Autodesk Inventor part; units mm, degrees
ref_plane "YZ Plane" through (0, 0, 0) normal (1, 0, 0) x (0, 1, 0)
ref_plane "XZ Plane" through (0, 0, 0) normal (0, 1, 0) x (-1, 0, 0)
ref_plane "XY Plane" through (0, 0, 0) normal (0, 0, 1) x (1, 0, 0)
sketch "Sketch1" plane through (0, 0, 0) normal (0, 1, 0) x (-1, 0, 0)
  line L0 (101.6, 38.1) -> (-101.6, 38.1) construction
  line L1 (-101.6, 38.1) -> (-101.6, -38.1) construction
  line L2 (-101.6, -38.1) -> (101.6, -38.1) construction
  line L3 (101.6, -38.1) -> (101.6, 38.1) construction
  line L4 (101.6, 38.1) -> (-101.6, -38.1) construction
  line L5 (-101.6, 38.1) -> (101.6, -38.1) construction
  line L6 (-28.575, 66.675) -> (28.575, 66.675) construction
  line L7 (28.575, 66.675) -> (28.575, 9.525)
  line L8 (28.575, 9.525) -> (-28.575, 9.525) construction
  line L9 (-28.575, 9.525) -> (-28.575, 66.675)
  line L10 (-28.575, 66.675) -> (28.575, 9.525) construction
  line L11 (28.575, 66.675) -> (-28.575, 9.525) construction
  circle A0 centre (-38.1, 50.8) radius 3.175
  line L12 (0, 38.1) -> (0, -38.1) construction
  circle A1 centre (-38.1, 50.8) radius 9.525
  line L13 (-38.1, 60.325) -> (-28.575, 60.325)
  circle A2 centre (38.1, 50.8) radius 3.175
  circle A3 centre (38.1, 50.8) radius 9.525
  line L14 (38.1, 60.325) -> (28.575, 60.325)
  circle A4 centre (-76.2, -38.1) radius 1.7526
  circle A5 centre (-95.25, 3.175) radius 1.7526
  circle A6 centre (76.2, -38.1) radius 1.7526
  circle A7 centre (95.25, 3.175) radius 1.7526
  line L15 (-101.6, -38.1) -> (-101.6, 6.35)
  line L16 (-101.6, 6.35) -> (-44.4797, 57.8728)
  line L17 (101.6, -38.1) -> (101.6, 6.35)
  line L18 (101.6, 6.35) -> (44.4797, 57.8728)
  line L19 (-42.6417, 42.4275) -> (-87.975, 1.5367) construction
  line L20 (-87.975, 1.5367) -> (-87.975, -38.1)
  line L21 (87.975, -38.1) -> (87.975, 1.5367)
  line L22 (87.975, 1.5367) -> (42.6417, 42.4275) construction
  line L23 (0, -38.1) -> (-95.25, -38.1) construction
  line L24 (0, -38.1) -> (95.25, -38.1) construction
  circle A8 centre (-60.325, 35.0287) radius 1.7526
  circle A9 centre (-33.3375, 31.75) radius 1.7526
  line L25 (-38.1, 0) -> (-38.1, 41.275)
  line L26 (-38.1, 0) -> (0, 0) construction
  circle A10 centre (60.325, 35.0287) radius 1.7526
  circle A11 centre (33.3375, 31.75) radius 1.7526
  line L27 (38.1, 0) -> (38.1, 41.275)
  line L28 (38.1, 0) -> (0, 0) construction
  line L29 (-87.975, 0) -> (-65.115, 0)
  line L30 (-65.115, 0) -> (-65.115, -31.75)
  line L31 (-65.115, -31.75) -> (-87.975, -31.75)
  line L32 (-101.6, -38.1) -> (101.6, -38.1) construction
  line L33 (101.6, -38.1) -> (101.6, 19.05)
  line L34 (101.6, 19.05) -> (-101.6, 19.05) construction
  line L35 (-101.6, 19.05) -> (-101.6, -38.1)
  line L36 (-101.6, 19.05) -> (-87.5203, 19.05) construction
  line L37 (87.5203, 19.05) -> (101.6, 19.05) construction
  circle A12 centre (-38.1, 0) radius 3.175 construction
  circle A13 centre (-38.1, 0) radius 6.35 construction
  circle A14 centre (38.1, 0) radius 3.175 construction
  circle A15 centre (38.1, 0) radius 6.35 construction
  circle A16 centre (28.575, 9.525) radius 1.7526
  circle A17 centre (28.575, 9.525) radius 4.7625
  arc A18 (17.0773, 9.525) -> (28.575, 21.0227) centre (17.0773, 21.0227) ccw
  circle A19 centre (-28.575, 9.525) radius 1.7526
  circle A20 centre (-28.575, 9.525) radius 4.7625
  arc A21 (-28.575, 21.0227) -> (-17.0773, 9.525) centre (-17.0773, 21.0227) ccw
  arc A22 (31.4325, 5.715) -> (38.1, 19.05) centre (21.4312, 19.05) ccw
  arc A23 (-38.1, 19.05) -> (-31.4325, 5.715) centre (-21.4312, 19.05) ccw
  line L38 (-61.94, -38.1) -> (-61.94, 25.0204)
  line L39 (87.975, 0) -> (65.115, 0)
  line L40 (65.115, 0) -> (65.115, -31.75)
  line L41 (65.115, -31.75) -> (87.975, -31.75)
  line L42 (61.94, -38.1) -> (61.94, 25.0204)
  line L43 (-28.575, 4.7625) -> (28.575, 4.7625)
  line L44 (101.6, -31.75) -> (-101.6, -31.75)
  line L45 (-101.6, -31.75) -> (-101.6, -44.45) construction
  line L46 (-101.6, -44.45) -> (101.6, -44.45)
  line L47 (101.6, -44.45) -> (101.6, -31.75) construction
  circle A24 centre (0, -38.1) radius 1.7526
  circle A25 centre (38.1, -38.1) radius 1.7526
  circle A26 centre (-38.1, -38.1) radius 1.7526
  line L48 (101.6, -38.1) -> (76.2, -44.45)
  line L49 (-101.6, -38.1) -> (-76.2, -44.45)
  line L50 (76.2, -38.1) -> (76.2, -44.45) construction
  line L51 (-76.2, -38.1) -> (-76.2, -44.45) construction
  line L52 (59.1924, 41.2769) -> (32.488, 36.4361)
  circle A27 centre (60.325, 35.0287) radius 6.35
  circle A28 centre (33.3375, 31.75) radius 4.7625
  line L53 (-59.1924, 41.2769) -> (-32.488, 36.4361)
  circle A29 centre (-60.325, 35.0287) radius 6.35
  circle A30 centre (-33.3375, 31.75) radius 4.7625
  line L54 (-87.975, 0) -> (-65.115, 0)
  line L55 (-65.115, 0) -> (-65.115, -3.175)
  line L56 (-65.115, -3.175) -> (-87.975, -3.175)
  line L57 (-87.975, -3.175) -> (-87.975, 0)
  line L58 (-65.115, -15.875) -> (-87.975, -15.875) construction
  line L59 (-65.115, -28.575) -> (-87.975, -28.575)
  line L60 (-84.8, -38.1) -> (-84.8, 0.1248)
  line L61 (65.115, -3.175) -> (87.975, -3.175)
  line L62 (65.115, -15.875) -> (87.975, -15.875) construction
  line L63 (65.115, -28.575) -> (87.975, -28.575)
  line L64 (84.8, -38.1) -> (84.8, 0.1248)
  line L65 (-33.3375, -31.75) -> (33.3375, -31.75)
  line L66 (33.3375, -31.75) -> (33.3375, 1.5875) construction
  line L67 (33.3375, 1.5875) -> (-33.3375, 1.5875)
  line L68 (-33.3375, 1.5875) -> (-33.3375, -31.75) construction
  circle A31 centre (41.275, 25.4) radius 3.175
  circle A32 centre (-41.275, 25.4) radius 3.175
  line L69 (-17.0773, 9.525) -> (17.0773, 9.525)
  line L70 (0, -31.75) -> (-41.275, -31.75)
  line L71 (-41.275, -31.75) -> (-33.3375, 1.5875)
  line L72 (41.275, -31.75) -> (33.3375, 1.5875)
  point P0 (28.575, 38.1)
  point P1 (-28.575, 38.1)
  point P2 (28.575, 60.325)
  point P3 (44.4797, 57.8728)
  point P4 (101.6, -15.875)
  point P5 (38.1, 41.275)
  point P6 (-87.975, -31.75)
  point P7 (-101.6, 6.35)
  point P8 (101.6, 6.35)
  point P9 (31.75, 0)
  point P10 (38.1, 6.35)
  point P11 (-38.1, 6.35)
  point P12 (-31.75, 0)
  point P13 (87.975, 0)
  point P14 (61.94, 25.0204)
  point P15 (-17.0773, 9.525)
  point P16 (-28.575, 21.0227)
  point P17 (-38.1, 19.05)
  point P18 (-31.4325, 5.715)
  point P19 (-21.8502, 0)
  point P20 (21.8502, 0)
  point P21 (-25.2074, 12.8926)
  point P22 (-28.575, 14.2875)
  point P23 (-23.8125, 9.525)
  point P24 (-28.575, 50.8)
  point P25 (25.2074, 12.8926)
  point P26 (28.575, 14.2875)
  point P27 (23.8125, 9.525)
  point P28 (28.575, 50.8)
  point P29 (26.8224, 9.525)
  point P30 (28.575, 11.2776)
  point P31 (61.94, -31.75)
  point P32 (-61.94, -31.75)
  point P33 (-28.575, 31.75)
  point P34 (-64.5781, 39.7439)
  point P35 (64.5781, 39.7439)
  point P36 (28.575, 31.75)
  point P37 (-84.8, -3.175)
  point P38 (-84.8, -28.575)
  point P39 (84.8, -3.175)
  point P40 (84.8, -28.575)
  point P41 (33.3375, -31.75)
  point P42 (-101.6, -31.75)
  point P43 (-26.8224, 9.525)
  point P44 (-28.575, 11.2776)
  point P45 (-39.8526, -38.1)
  point P46 (-36.3474, -38.1)
  point P47 (-1.7526, -38.1)
  point P48 (1.7526, -38.1)
  point P49 (36.3474, -38.1)
  point P50 (39.8526, -38.1)
  point P51 (41.275, -31.75)
  dimension "d0" = 203.2
  dimension "d1" = 76.2
  dimension "d4" = 57.15
  dimension "d6" = 6.35
  dimension "d7" = 38.1
  dimension "d8" = 19.05
  dimension "d10" = 3.5052
  dimension "d11" = 3.5052
  dimension "d12" = 0
  dimension "d14" = 25.4
  dimension "d15" = 6.35
  dimension "d20" = 50.8
  dimension "d21" = 41.275
  dimension "d22" = 44.45
  dimension "d24" = 12.7
  dimension "d25" = 13.625
  dimension "d26" = 12.7
  dimension "d27" = 13.625
  dimension "d31" = 3.5052
  dimension "d32" = 3.5052
  dimension "d33" = 6.35
  dimension "d34" = 31.75
  dimension "d35" = 4.7625
  dimension "d36" = 22.225
  dimension "d37" = 9.525
  dimension "d39" = 31.75
  dimension "d40" = 6.35
  dimension "d42" = 57.15
  dimension "d43" = 6.35
  dimension "d44" = 9.525
  dimension "d45" = 9.525
  dimension "d46" = 12.7
  dimension "d104" = 3.5052
  dimension "d105" = 9.525
  dimension "d106" = 3.175
  dimension "d107" = 22.86
  dimension "d123" = 88.9
  dimension "d124" = 12.7
  dimension "d125" = 3.5052
  dimension "d126" = 3.5052
  dimension "d127" = 38.1
  dimension "d128" = 28.575
  dimension "d129" = 3.175
  dimension "d130" = 3.175
  dimension "d131" = 33.3375
  dimension "d132" = 33.3375
  dimension "d133" = 33.3375
  dimension "d135" = 6.35
  dimension "d138" = 6.35
  dimension "d139" = 3.175
  dimension "d140" = 41.275
extrude "Extrusion1" add sketch "Sketch1" along normal blind 3.175 contours A28 L27 A22 A17 L7 | A28 | L7 A17 A18 | L52 L27 A28 | L27 L52 A27 L18 L17 L44 L21 L39 L40 L72 L67 L71 L30 L29 L20 L15 L16 A29 L53 L25 A23 A20 L43 A17 A22 | A27 | A17 | A17 L43 A20 A21 L69 A18 | L17 L48 L46 L49 L15 L44 L31 L41 | A20 | L41 L64 L63 L21 | A23 L25 A30 L9 A20 | A20 L9 A21 | L63 L64 L61 L21 | L41 L40 L63 L64 | L61 L64 L39 L21 | A30 | L61 L40 L39 L64 | L25 L53 A30 | L20 L59 L60 L31 | A29 | L20 L56 L60 L59 | L60 L59 L30 L31 | L20 L29 L60 L56 | L60 L29 L30 L56
fillet "Fillet1" radius 6.35 14 edges at (101.6, 1.5875, -38.1) (101.6, 1.5875, 6.35) (-101.6, 1.5875, 6.35) (76.2, 1.5875, -44.45) (-76.2, 1.5875, -44.45) (-101.6, 1.5875, -38.1) (-84.8, 1.5875, -28.575) (-84.8, 1.5875, -3.175) (-65.115, 1.5875, -28.575) (-65.115, 1.5875, -3.175) (65.115, 1.5875, -28.575) (84.8, 1.5875, -28.575) (84.8, 1.5875, -3.175) (65.115, 1.5875, -3.175)
fillet "Fillet5" radius 6.35 4 edges at (33.3375, 1.5875, 1.5875) (-33.3375, 1.5875, 1.5875) (-41.275, 1.5875, -31.75) (41.275, 1.5875, -31.75)
equation "\"d35\" = 0.5 * d37"
properties part number "Chassis" material "UHMW, Black"
Verification items for the finished model (mm, model axes). A direction names the side the tool comes from. Give positions to 0.01 mm unless a question says otherwise; leave off trailing zeros. Order: outer loops, then holes, each group sorted by start corner. A loop starts at its lowest first (then second) coordinate and runs counter-clockwise, first axis right, second up. Notation, with made-up numbers: M 17,57.5 L 45,57.5 A23 cw 45,69.5 Z; hole C 25,14 d6. An arc over 180 degrees is marked long. Use one line per item in the form item = value. Start each with the question number.
Q1. Section check A-A (z = -19). Enter the section's corners in (x, y) (3 decimals).
Q2. Go/stop test with flat-tipped pins: pin 1 Ø3 at (x, z) = (73.5, -6) entering from -Y; pin 2 Ø1 at (x, y) = (-53, 2) entering from +Z (3 decimals). Record where each tip stops, or that it passes through.
Q3. Scan lines: line 1 along X through (y, z) = (2.35, -17) (3 decimals); line 2 along Z through (x, y) = (29, 2.25); line 3 along X through (y, z) = (1.5, 23) (3 decimals). Record each from-to range of solid material in increasing order. Write a range as [from, to].
Q4. Mould release check, pull along X, two halves, no side actions. Record for faces 4 (the flat face through (82.29, 1.57, 23.77)), 5 (the flat face through (-87.013, 1.565, -41.747)), 6 (the cylindrical face through (-34.956, 1.565, 32.421)): +X half, -X half, draft (parallel to the pull), parting line (faces both ways), or undercut.
Q5. Section check B-B (x = 82.5). Enter the section's corners in (y, z) (3 decimals), then the cut area to 3 significant figures.
Q6. Section check C-C (z = 17). Enter the section's corners in (x, y) (3 decimals).
Q7. Section check D-D (y = 1.2). Count the separate pieces of the cut face and the enclosed holes in it, then the cut area to 3 significant figures.
Q8. Access from +Z, -Z, +X, -X, +Y, -Y to the whole of each face (thin tool, end or side, straight path). Record for faces 1 (the flat face through (37, 1.6, -13.8)), 2 (the flat face through (-82.29, 1.57, 23.77)), 3 (the cylindrical face through (29.712, 1.565, 34.838)).
Evaluation:
q1.outline = M -101.6,0 L -84.8,0 L -84.8,3.175 L -101.6,3.175 Z; M -65.115,0 L -38.239,0 L -38.239,3.175 L -65.115,3.175 Z; M 38.239,0 L 65.115,0 L 65.115,3.175 L 38.239,3.175 Z; M 84.8,0 L 101.6,0 L 101.6,3.175 L 84.8,3.175 Z
q2.pin_1 = through
q2.pin_2 = 40.245
q3.line_1 = [-101.6, -84.8], [-65.115, -37.763], [37.763, 65.115], [84.8, 101.6]
q3.line_2 = [-44.45, -31.75], [1.55, 7.82], [11.23, 33.72]
q3.line_3 = [-83.141, -43.354], [-39.196, -28.575], [28.575, 39.196], [43.354, 83.141]
q4.face_4 = +X half
q4.face_5 = -X half
q4.face_6 = undercut
q5.outline = M 0,-42.875 L 3.175,-42.875 L 3.175,-27.116 L 0,-27.116 Z; M 0,-4.634 L 3.175,-4.634 L 3.175,23.578 L 0,23.578 Z
q5.area = 140 mm2
q6.outline = M -89.793,0 L -27.848,0 L -27.848,3.175 L -89.793,3.175 Z; M 27.848,0 L 89.793,0 L 89.793,3.175 L 27.848,3.175 Z
q7.separate_pieces = 1
q7.enclosed_holes = 18
q7.area = 10,400 mm2
q8.face_1 = +Y, -Y
q8.face_2 = +Z, -X, +Y, -Y
q8.face_3 = +Z, +Y, -Y
